Print and shaded views of the part. All mm, measured from the part's lowest x, y and z. A direction names the side the tool comes from. Coordinates: 2 decimals unless noted, no trailing zeros. Order: outer loops, then holes, each group sorted by start corner. A loop starts at its lowest first (then second) coordinate and runs counter-clockwise, first axis right, second up. Notation, with made-up numbers: (30.5, -9) - (34.5, -9) arc R29 cw to (34.5, 22) - close; hole circle Ø5 at (11, -26.75). An arc over 180 degrees is marked (long way). Write each question's results on one line, items separated by ' | '.
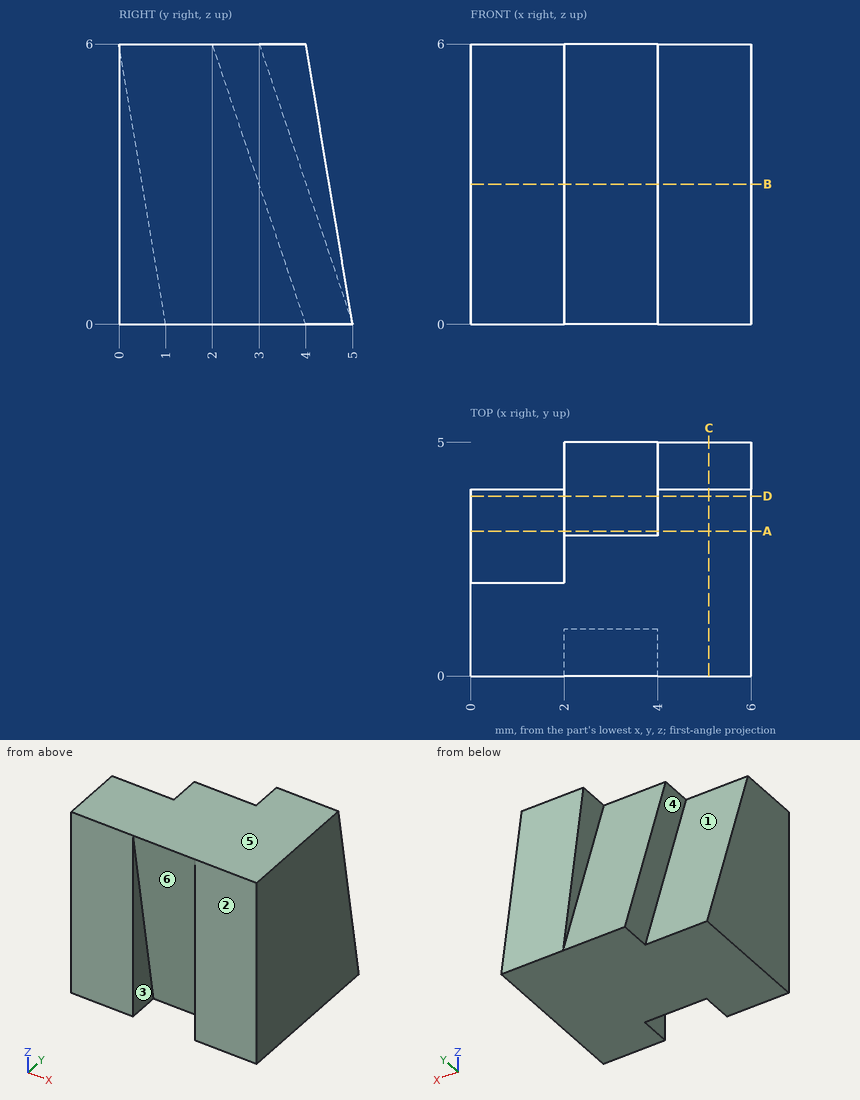
1. Band-saw the part on B-B on z = 3. Give the cut face in (x, y).
Solved:
outline: (0, 0) - (2, 0) - (2, 0.5) - (4, 0.5) - (4, 0) - (6, 0) - (6, 4.5) - (4, 4.5) - (4, 4) - (2, 4) - (2, 3) - (0, 3) - close
2. Band-saw the part on A-A on y = 3.1. Give the cut face in (x, z).
Solved:
outline: (0, 0) - (6, 0) - (6, 6) - (4, 6) - (4, 5.7) - (2, 5.7) - (2, 2.7) - (0, 2.7) - close
3. Drop flat-ended pins along their axis: pin 1 Ø0.9 at (y, z) = (4, 2.5) entering from -X; pin 2 Ø1 at (y, z) = (4, 5) entering from -X. Give the stop position or say it passes through.
Solved:
pin 1: stops at x = 2 | pin 2: stops at x = 4
4. Band-saw the part on C-C on x = 5.1. Give the cut face in (y, z).
Solved:
outline: (0, 0) - (5, 0) - (4, 6) - (0, 6) - close
5. Band-saw the part on D-D on y = 3.85. Give the cut face in (x, z).
Solved:
outline: (0, 0) - (6, 0) - (6, 6) - (4, 6) - (4, 3.45) - (2, 3.45) - (2, 0.45) - (0, 0.45) - close
6. Tool access for the marked faces 1, 2 and 3: list every direction of +Z, -Z, +X, -X, +Y, -Y with a clear straight run to the whole face (end or side of a thin tool).
Solved:
face 1: +Z, -X, +Y | face 2: +Z, -Z, +X, -X, -Y | face 3: -Z, -Y
7. Two-plate mould, pull along X, no slides. Class the marked faces 4, 5 and 6: +X half, -X half, draft (parallel to the pull), parting line (faces both ways), or undercut.
Solved:
face 4: -X half | face 5: draft | face 6: undercut
8. Probe line 1 (X direction, y = 3.1, z = 3); line 2 (Y direction, x = 2.7, z = 3.5); line 3 (Y direction, x = 1.8, z = 4). List the from-to ranges inside material, lowest first.
Solved:
line 1: x = 2 to 6 | line 2: y = 0.42 to 3.83 | line 3: y = 0 to 2.67
